Part model, mm, in its own coordinate system. A direction names the side the tool comes from. Give positions to 0.01 mm unless a question says otherwise; leave off trailing zeros. Answer as a JSON object with one key per item and string values.
Autodesk Inventor part; units mm, degrees
ref_plane "YZ Plane" through (0, 0, 0) normal (1, 0, 0) x (0, 1, 0)
ref_plane "XZ Plane" through (0, 0, 0) normal (0, 1, 0) x (-1, 0, 0)
ref_plane "XY Plane" through (0, 0, 0) normal (0, 0, 1) x (1, 0, 0)
sketch "Skizze1" plane through (0, 0, 0) normal (0, 0, 1) x (1, 0, 0)
  line L0 (38, -12.9) -> (-38, -12.9)
  line L1 (-38, -12.9) -> (-38, 12.9)
  line L2 (-38, 12.9) -> (38, 12.9)
  line L3 (38, 12.9) -> (38, -12.9)
  line L4 (38, -12.9) -> (-38, 12.9) construction
  line L5 (-38, -12.9) -> (38, 12.9) construction
  point P0 (0, 0)
  dimension "d0" = 76
  dimension "d1" = 25.8
extrude "Extrusion1" add sketch "Skizze1" along normal blind 4
sketch "Skizze2" plane through (0, 0, 4) normal (0, 0, 1) x (1, 0, 0)
  line L0 (38, 12.9) -> (-38, 12.9)
  line L1 (-38, 12.9) -> (-38, -12.9)
  line L2 (-38, -12.9) -> (38, -12.9)
  line L3 (38, -12.9) -> (38, 12.9)
  line L4 (2.5, -7.1) -> (-2.5, -7.1)
  line L5 (-2.5, -7.1) -> (-2.5, 12.9)
  line L6 (-2.5, 12.9) -> (2.5, 12.9)
  line L7 (2.5, 12.9) -> (2.5, -7.1)
  line L8 (2.5, -7.1) -> (-2.5, 12.9) construction
  line L9 (-2.5, -7.1) -> (2.5, 12.9) construction
  point P0 (0, 0)
  point P1 (0, 2.9)
  point P2 (0, 12.9)
  dimension "d4" = 5
  dimension "d5" = 20
extrude "Extrusion2" cut sketch "Skizze2" against normal blind 1.5 contours L7 L4 L5 L0
sketch "Skizze3" plane through (-38, 12.9, 0) normal (0, 1, 0) x (1, 0, 0)
  line L0 (40.5, -4) -> (35.5, -4)
  line L1 (40.5, -4) -> (40.5, -2.5)
  line L2 (40.5, -2.5) -> (35.5, -2.5)
  line L3 (35.5, -4) -> (35.5, -2.5)
  circle A0 centre (38, -3.875) radius 0.125
  point P0 (38, 0)
  dimension "d8" = 0.25
extrude "Extrusion3" add sketch "Skizze3" against normal up to surface (20 mm away) contours A0
pattern_linear "Rechteckige Anordnung1" count 11 spacing 0.25 along (-1, 0, 0) count 11 spacing 0.25 along (1, 0, 0) of "Extrusion3"
ref_plane "Arbeitsebene1" through (0, -12.9, 0) normal (1, 0, 0) x (0, 0, -1)
properties part number "00_chipnano_waveguide_slidsize"
1. Two-plate mould, pull along X, no slides. Class faces 1 (the flat face through (0, -7.1, 3)), 2 (the flat face through (0, 3, 2.5)), 3 (the flat face through (38, 0, 2)), 4 (the flat face through (1, -12.9, 2)): +X half, -X half, draft (parallel to the pull), parting line (faces both ways), or undercut.
Worked answers:
{"face 1": "undercut", "face 2": "undercut", "face 3": "+X half", "face 4": "draft"}
2. Probe line 1 along X through (y, z) = (6, 3.3). List the from-to ranges inside material, lowest first.
Worked answers:
{"line 1": "x = -38 to -2.5, 2.5 to 38"}
3. Which spindle directions (+Z, -Z, +X, -X, +Y, -Y) get a long thin tool onto all of the face, cutting with end or side? Do faces 5 (the flat face through (-1, 0, 0)), 6 (the flat face through (2.5, 3, 3)). Say none if no direction does.
Worked answers:
{"face 5": "-Z, +X, -X, +Y, -Y", "face 6": "+Y"}
